The listing builds one solid part. Answer for the finished solid, in the listing's coordinates (mm). A direction names the side the tool comes from. Coordinates: 2 decimals unless noted, no trailing zeros. Order: outer loops, then holes, each group sorted by start corner. A loop starts at its lowest first (then second) coordinate and runs counter-clockwise, first axis right, second up. Notation, with made-up numbers: (64.5, -36.75) -> (80.5, -36.75) arc R8 cw to (80.5, -27.75) -> close; hole circle Ø2 at (12, 37.5). An arc over 180 degrees is marked (long way). Write item = value, one per line. Start each with the question number.
```python
from build123d import *

# Parameters (mm, degrees)
SKETCH1_R               = 3.25
SKETCH1_W               = 10
SKETCH1_H               = 26.165
SKETCH1_H_2             = 10.835
SKETCH1_H_3             = 13
SKETCH1_H_4             = 5
BOSS_EXTRUDE2_DEPTH     = 5
SKETCH1_6_W             = 10
SKETCH1_6_H             = 10.835
SKETCH1_6_H_2           = 5
BOSS_EXTRUDE3_DEPTH     = 30
CUT_EXTRUDE1_DEPTH      = 59.303623387
CUT_EXTRUDE1_DEPTH_BACK = 59.303623387
SKETCH4_R               = 1.75
SKETCH3_R               = 1.75
CUT_EXTRUDE2_DEPTH      = 59.303623387


with BuildPart() as part:
    # Sketch1 → Boss-Extrude2 (new body)
    # profile 1 of 5: a face of its own
    with BuildSketch(Plane(origin=(0, 0, 0), x_dir=(1, 0, 0), z_dir=(0, 1, 0))):
        Polygon((28.25, 27.5), (-13.5, 27.5), (-13.5, 16.665), (-13.5, -9.5), (-13.5, -14.5), (-13.5, -27.5), (28.25, -27.5), align=None)
        with Locations(Location((-6.75, -16.665, 0), (0, 0, 270))):
            Circle(SKETCH1_R, mode=Mode.SUBTRACT)
        with Locations(Location((18.25, -16.665, 0), (0, 0, 270))):
            Circle(SKETCH1_R, mode=Mode.SUBTRACT)
        with Locations(Location((-6.75, 16.665, 0), (0, 0, 270))):
            Circle(SKETCH1_R, mode=Mode.SUBTRACT)
        with Locations(Location((18.25, 16.665, 0), (0, 0, 270))):
            Circle(SKETCH1_R, mode=Mode.SUBTRACT)
    # profile 2 of 5: a face of its own
    with BuildSketch(Plane(origin=(0, 0, 0), x_dir=(1, 0, 0), z_dir=(0, 1, 0))):
        with Locations((-18.5, 3.5825)):
            Rectangle(SKETCH1_W, SKETCH1_H)
    # profile 3 of 5: a face of its own
    with BuildSketch(Plane(origin=(0, 0, 0), x_dir=(1, 0, 0), z_dir=(0, 1, 0))):
        with Locations((-18.5, 22.0825)):
            Rectangle(SKETCH1_W, SKETCH1_H_2)
    # profile 4 of 5: a face of its own
    with BuildSketch(Plane(origin=(0, 0, 0), x_dir=(1, 0, 0), z_dir=(0, 1, 0))):
        with Locations((-18.5, -21)):
            Rectangle(SKETCH1_W, SKETCH1_H_3)
    # profile 5 of 5: a face of its own
    with BuildSketch(Plane(origin=(0, 0, 0), x_dir=(1, 0, 0), z_dir=(0, 1, 0))):
        with Locations((-18.5, -12)):
            Rectangle(SKETCH1_W, SKETCH1_H_4)
    extrude(amount=BOSS_EXTRUDE2_DEPTH)

    # Sketch1_6 → Boss-Extrude3 (add)
    with BuildSketch(Plane(origin=(0, 0, 0), x_dir=(1, 0, 0), z_dir=(0, 1, 0))):
        with Locations((-18.5, 22.0825)):
            Rectangle(SKETCH1_6_W, SKETCH1_6_H)
        with Locations((-18.5, -12)):
            Rectangle(SKETCH1_6_W, SKETCH1_6_H_2)
    extrude(amount=BOSS_EXTRUDE3_DEPTH)

    # Sketch4 → Cut-Extrude1 (cut, two sides: drawn at the far end of the back side and taken through both)
    with BuildSketch(Plane(origin=(-13.5, 0, 0), x_dir=(0, 0, -1), z_dir=(1, 0, 0)).offset(-CUT_EXTRUDE1_DEPTH_BACK)):
        with Locations((22.0825, 26.25)):
            Circle(SKETCH4_R)
        with Locations((22.0825, 8.75)):
            Circle(SKETCH4_R)
    extrude(amount=CUT_EXTRUDE1_DEPTH + CUT_EXTRUDE1_DEPTH_BACK, mode=Mode.SUBTRACT)

    # Sketch3 → Cut-Extrude2 (cut, through all)
    with BuildSketch(Plane(origin=(-13.5, 0, 0), x_dir=(0, 0, -1), z_dir=(1, 0, 0))):
        with Locations((-12, 17.5)):
            Circle(SKETCH3_R)
    extrude(amount=-CUT_EXTRUDE2_DEPTH, mode=Mode.SUBTRACT)


solid = part.part
```
Item 1: Each of these flat-tipped pins is pushed along its axis until it touches: pin 1 (2.5 mm diameter, centred on y = 21.5, z = 12, fed in from +X); pin 2 (8 mm diameter, centred on x = -14.5, z = -10.5, fed in from +Y); pin 3 (8 mm diameter, centred on x = -18.5, y = 17.5, fed in from +Z). Where does it stop, or does it pass through?
Item 2: Consider probe 1 along Z at (x, y) = (-16.5, 8.75) (1 decimal); probe 2 along Z at (x, y) = (-14, 16) (3 decimals); probe 3 along X at (y, z) = (2.5, -15). Determine where each line is inside the solid, lowest interval first.
Item 3: Which of the six approach directions +Z, -Z, +X, -X, +Y, -Y give full straight-line access (tool end or side, diameter ignored) to faces 4 (the flat face through (-19, 17, 14.5)), 5 (the flat face through (-13.5, 17, -22)), 6 (the flat face through (-19, 17, -16.665)), 7 (the cylindrical face through (-18.43, 19.235, 12.228))?
Item 4: Section C-C, the plane x = -6.75 is taken. Give the vertices of the cut face in (y, z) (3 decimals), then the cut area to 3 significant figures.
Item 5: For a pull along Y with two mould halves and no side action, classify faces 1 (the flat face through (28.25, 2, 0)), 2 (the cylindrical face through (-18.57, 8.827, -20.334)), 3 (the flat face through (-19, 30, 12)) as pulls with the +Y half, pulls with the -Y half, needs draft (parallel to the pull), parting line crosses it, or undercut.
Item 6: Section D-D, the plane y = 26.25 is taken. Give the vertices of the cut face in (x, z) (1 decimal), then the cut area to 3 significant figures.
Item 7: Section B-B, the plane z = 12 is taken. Give the vertices of the cut face in (x, y).
Item 8: Section A-A, the plane y = 11.5 is taken. Give the vertices of the cut face in (x, z) (3 decimals), then the cut area to 3 significant figures.
A:
q1.pin_1 = -13.5
q1.pin_2 = 5
q1.pin_3 = 14.5
q2.probe_1 = -27.5 to -23.8, -20.3 to -16.7, 9.5 to 14.5
q2.probe_2 = -27.5 to -16.665, 9.5 to 11.099, 12.901 to 14.5
q2.probe_3 = -23.5 to -9.54, -3.96 to 15.46, 21.04 to 28.25
q3.face_4 = +Z, +X, -X, +Y
q3.face_5 = +Z, -Z, +X, +Y
q3.face_6 = +X, -X, +Y
q3.face_7 = +X, -X
q4.outline = (0, -27.5) -> (5, -27.5) -> (5, -19.915) -> (0, -19.915) -> close; (0, -13.415) -> (5, -13.415) -> (5, 13.415) -> (0, 13.415) -> close; (0, 19.915) -> (5, 19.915) -> (5, 27.5) -> (0, 27.5) -> close
q4.area = 210 mm^2
q5.face_1 = needs draft
q5.face_2 = undercut
q5.face_3 = pulls with the +Y half
q6.outline = (-23.5, -27.5) -> (-13.5, -27.5) -> (-13.5, -23.8) -> (-23.5, -23.8) -> close; (-23.5, -20.3) -> (-13.5, -20.3) -> (-13.5, -16.7) -> (-23.5, -16.7) -> close; (-23.5, 9.5) -> (-13.5, 9.5) -> (-13.5, 14.5) -> (-23.5, 14.5) -> close
q6.area = 123 mm^2
q7.outline = (-23.5, 0) -> (28.25, 0) -> (28.25, 5) -> (-13.5, 5) -> (-13.5, 15.75) -> (-23.5, 15.75) -> close; (-23.5, 19.25) -> (-13.5, 19.25) -> (-13.5, 30) -> (-23.5, 30) -> close
q8.outline = (-23.5, -27.5) -> (-13.5, -27.5) -> (-13.5, -16.665) -> (-23.5, -16.665) -> close; (-23.5, 9.5) -> (-13.5, 9.5) -> (-13.5, 14.5) -> (-23.5, 14.5) -> close
q8.area = 158 mm^2
